```python
from build123d import *

# Parameters (mm, degrees)
SKETCH1_W           = 164
SKETCH1_H           = 126
SKETCH1_R           = 4
BOSS_EXTRUDE1_DEPTH = 6
FILLET1_R           = 10
SKETCH2_R           = 2
SKETCH2_W           = 19.7
SKETCH2_H           = 29.7
CUT_EXTRUDE1_DEPTH  = 207.900942482


with BuildPart() as part:
    # Sketch1 → Boss-Extrude1 (new body)
    with BuildSketch(Plane(origin=(0, 0, 0), x_dir=(1, 0, 0), z_dir=(0, 1, 0))):
        with Locations((-82, 63)):
            Rectangle(SKETCH1_W, SKETCH1_H)
        with Locations(Location((-132.75, 107, 0), (0, 0, 270))):
            Circle(SKETCH1_R, mode=Mode.SUBTRACT)
        with Locations(Location((-31.25, 107, 0), (0, 0, 270))):
            Circle(SKETCH1_R, mode=Mode.SUBTRACT)
        with Locations(Location((-132.75, 19, 0), (0, 0, 270))):
            Circle(SKETCH1_R, mode=Mode.SUBTRACT)
        with Locations(Location((-31.25, 19, 0), (0, 0, 270))):
            Circle(SKETCH1_R, mode=Mode.SUBTRACT)
    extrude(amount=BOSS_EXTRUDE1_DEPTH)

    # Fillet1
    fillet1_edges = [part.edges().sort_by_distance(p)[0] for p in [
        (0, 3, 0),
        (-164, 3, 0),
        (-164, 3, -126),
        (0, 3, -126),
    ]]
    fillet(fillet1_edges, radius=FILLET1_R)

    # Sketch2 → Cut-Extrude1 (cut, through all)
    with BuildSketch(Plane(origin=(0, 6, 0), x_dir=(1, 0, 0), z_dir=(0, 1, 0))):
        with Locations(Location((-88.25, 84, 0), (0, 0, 270))):
            Circle(SKETCH2_R)
        with Locations(Location((-75.75, 84, 0), (0, 0, 270))):
            Circle(SKETCH2_R)
        with Locations(Location((-98, 69.75, 0), (0, 0, 270))):
            Circle(SKETCH2_R)
        with Locations(Location((-98, 56.25, 0), (0, 0, 270))):
            Circle(SKETCH2_R)
        with Locations(Location((-88.25, 42, 0), (0, 0, 270))):
            Circle(SKETCH2_R)
        with Locations(Location((-75.75, 42, 0), (0, 0, 270))):
            Circle(SKETCH2_R)
        with Locations(Location((-66, 56.25, 0), (0, 0, 270))):
            Circle(SKETCH2_R)
        with Locations(Location((-66, 69.75, 0), (0, 0, 270))):
            Circle(SKETCH2_R)
        with Locations((-82, 63)):
            Rectangle(SKETCH2_W, SKETCH2_H)
    extrude(amount=-CUT_EXTRUDE1_DEPTH, mode=Mode.SUBTRACT)


solid = part.part
```
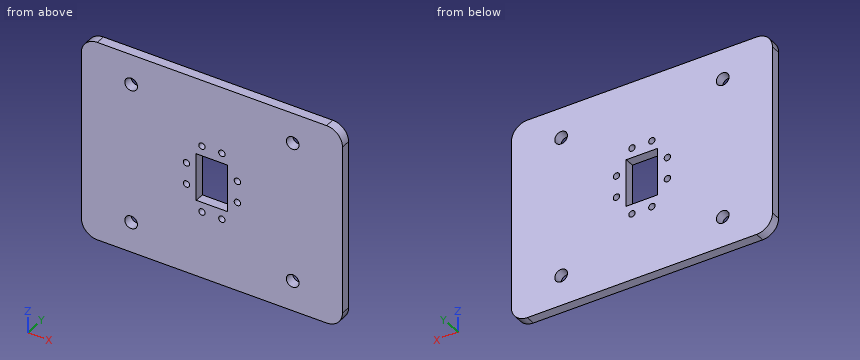
Here's how the part is built. I have some questions about the finished solid (model axes, mm). Coordinates: 2 decimals unless noted, no trailing zeros. Write each loop counter-clockwise with the first axis right and the second up, starting at its lowest first coordinate (ties: lowest second). Pieces come first, ordered by that corner, then holes. Notation, with made-up numbers: M 51.5,5.25 L 57.5,5.25 A8 ccw 57.5,14.25 Z; hole C -29,-8.75 d7. An arc over 180 degrees is marked long. Answer as CSV lines item,"result". Start each with the question number.
Q1. Suppose I cut it at B-B, the plane z = -69.75. List the corners of the cut face in (x, y) for me.
Q2. Will this pin go through, and if not, where does the flat tip stop? pin 1 Ø6.5 at (x, z) = (-31.25, -107) entering from +Y.
Q3. Suppose I cut it at C-C, the plane y = 4.9. State how many separate pieces and enclosed holes the cut face has, then the cut area to 3 significant figures.
Q4. Suppose I cut it at A-A, the plane x = -66. List the corners of the cut face in (y, z) for me, then the cut area to 3 significant figures.
Q5. Suppose I cut it at D-D, the plane z = -107. List the corners of the cut face in (x, y) for me, then the cut area to 3 significant figures.
Q6. I need wall thicknesses on probe 1 along X at (y, z) = (2.5, -42); probe 2 along X at (y, z) = (1.95, -107); probe 3 along X at (y, z) = (2.25, -69.75). Which ranges of each line are inside material? Lowest first, please. Write a range as [from, to].
Entries:
1,outline,"M -164,0 L -100,0 L -100,6 L -164,6 Z; M -96,0 L -91.85,0 L -91.85,6 L -96,6 Z; M -72.15,0 L -68,0 L -68,6 L -72.15,6 Z; M -64,0 L 0,0 L 0,6 L -64,6 Z"
2,pin 1,"passes through"
3,separate pieces,"1"
3,enclosed holes,"13"
3,area,"19,700 mm²"
4,outline,"M 0,-126 L 6,-126 L 6,-71.75 L 0,-71.75 Z; M 0,-67.75 L 6,-67.75 L 6,-58.25 L 0,-58.25 Z; M 0,-54.25 L 6,-54.25 L 6,0 L 0,0 Z"
4,area,"708 mm²"
5,outline,"M -164,0 L -136.75,0 L -136.75,6 L -164,6 Z; M -128.75,0 L -35.25,0 L -35.25,6 L -128.75,6 Z; M -27.25,0 L 0,0 L 0,6 L -27.25,6 Z"
5,area,"888 mm²"
6,probe 1,"x = [-164, -90.25], [-86.25, -77.75], [-73.75, 0]"
6,probe 2,"x = [-164, -136.75], [-128.75, -35.25], [-27.25, 0]"
6,probe 3,"x = [-164, -100], [-96, -91.85], [-72.15, -68], [-64, 0]"
